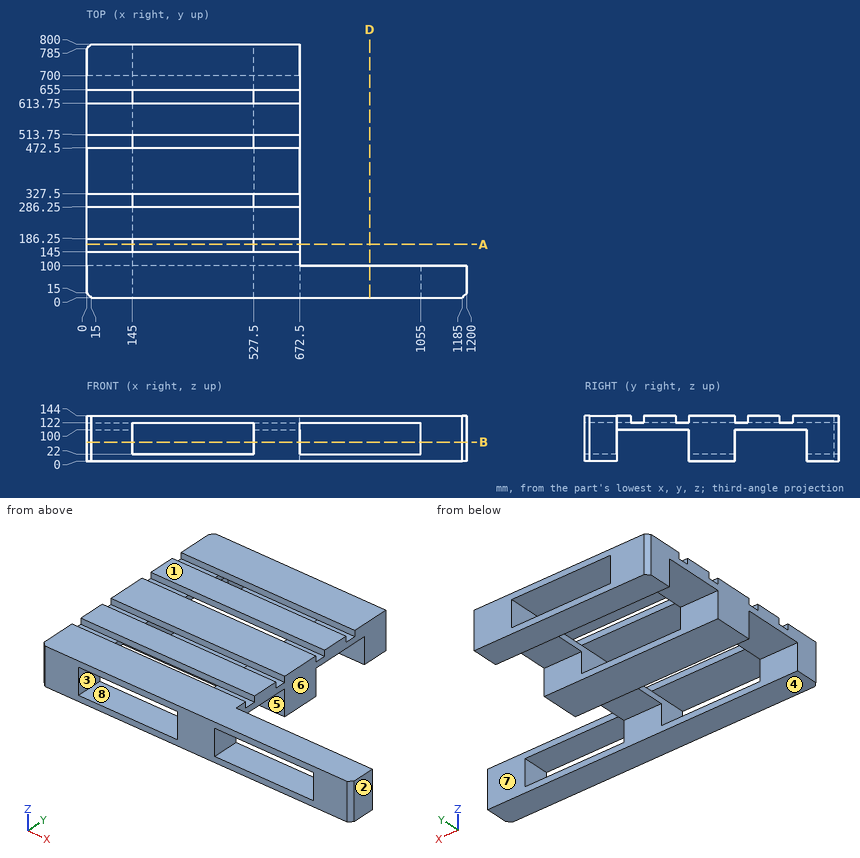
Geometry check sheet. Reference: drawing and pictorial views, mm from the part's lowest x, y, z. A direction names the side the tool comes from. Give positions to 0.01 mm unless a question says otherwise; leave off trailing zeros. Order: outer loops, then holes, each group sorted by start corner. A loop starts at its lowest first (then second) coordinate and runs counter-clockwise, first axis right, second up. Notation, with made-up numbers: (59, -8.5) - (75, -8.5) arc R13 ccw to (75, -0.5) - close; hole circle Ø2 at (67.25, 1). An arc over 180 degrees is marked (long way). Answer as CSV lines item,"result". Start each with the question number.
Item 1: Mould release check, pull along X, two halves, no side actions. Record for the marked faces 1, 2 and 3: released by +X, released by -X, zero draft, split by the parting line, or undercut.
Item 2: Section check A-A, the plane y = 168. Record the boundary of the cut face in (x, z).
Item 3: Section check D-D, the plane x = 893. Record the boundary of the cut face in (y, z).
Item 4: Material ranges on L1, parallel to X at y = 47, z = 84.5; L2, parallel to Y at x = 554, z = 31; L3, parallel to Y at x = 661, z = 128.5, recorded low to high.
Item 5: Gauge pin test, flat ends, axial feed: pin 1 (1 mm diameter, centred on x = 442, y = 611.5, fed in from -Z); pin 2 (2 mm diameter, centred on y = 700.5, z = 100.5, fed in from +X); pin 3 (12.5 mm diameter, centred on x = 601, y = 160, fed in from +Z). Record the tip position at first contact, or that the pin passes through.
Item 6: Section check B-B, the plane z = 60. State how many separate pieces and enclosed holes the cut face has, plus the area to 3 significant figures.
Item 7: Access from +Z, -Z, +X, -X, +Y, -Y to the whole of each face (thin tool, end or side, straight path). Record for the marked faces 4, 5, 6, 7 and 8.
Filled in:
1,face 1,"zero draft"
1,face 2,"released by +X"
1,face 3,"undercut"
2,outline,"(0, 100) - (145, 100) - (145, 122) - (0, 122) - close; (527.5, 100) - (672.5, 100) - (672.5, 122) - (527.5, 122) - close"
3,outline,"(0, 0) - (100, 0) - (100, 22) - (0, 22) - close; (0, 122) - (100, 122) - (100, 144) - (0, 144) - close"
4,L1,"0 to 145, 527.5 to 672.5, 1055 to 1200"
4,L2,"0 to 100, 327.5 to 472.5, 700 to 800"
4,L3,"0 to 145, 186.25 to 286.25, 327.5 to 472.5, 513.75 to 613.75, 655 to 800"
5,pin 1,"z = 122"
5,pin 2,"x = 672.5"
5,pin 3,"z = 122"
6,separate pieces,"7"
6,enclosed holes,"0"
6,area,"114,000 mm^2"
7,face 4,"-Z, +X, -X, +Y, -Y"
7,face 5,"-Z, +X, -X"
7,face 6,"+Y"
7,face 7,"-Z, +X"
7,face 8,"+Y, -Y"
